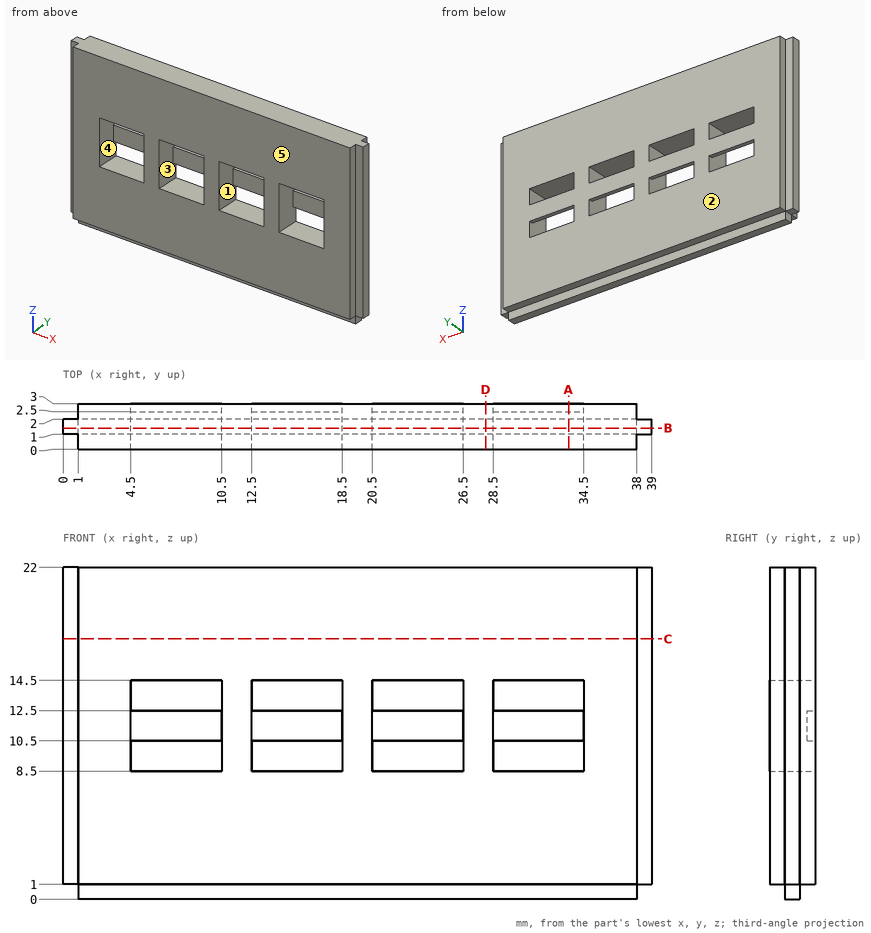
Here's the drawing with two shaded views (mm, measured from the low corner). I have some questions. A direction names the side the tool comes from. Coordinates: 2 decimals unless noted, no trailing zeros. Order: outer loops, then holes, each group sorted by start corner. A loop starts at its lowest first (then second) coordinate and runs counter-clockwise, first axis right, second up.
Q1. Suppose I cut it at C-C on z = 17.25. Please give me the cut outline in (x, y).
Q2. Which directions (+Z, -Z, +X, -X, +Y, -Y) give clear straight access to the entire face, cutting with the end or side of a thin tool? Please do the marked faces 4 and 5.
Q3. Suppose I cut it at B-B on y = 1.4. Please give me the cut outline in (x, z).
Q4. Please list where these lines run through material, in increasing order: L1, parallel to X at y = 1.4, z = 12; L2, parallel to Z at x = 30, y = 2.2; L3, parallel to Z at x = 34, y = 1.3.
Q5. Thinking about a two-plate mould opening in X: for the marked faces 1, 2 and 3, which applies, released by +X, released by -X, zero draft, split by the parting line, or undercut?
Q6. Will these pins go through, and if not, where does the flat tip stop? pin 1 (1.6 mm diameter, centred on x = 6.5, z = 11.5, fed in from -Y); pin 2 (0.6 mm diameter, centred on x = 8.5, y = 3, fed in from -Z); pin 3 (0.8 mm diameter, centred on y = 0.5, z = 12, fed in from +X).
Q7. Suppose I cut it at A-A on x = 33.5. Please give me the cut outline in (y, z).
Q8. Suppose I cut it at D-D on x = 28. Please give me the cut outline in (y, z).
Answer:
1. outline: (0, 1) - (1, 1) - (1, 0) - (38, 0) - (38, 1) - (39, 1) - (39, 2) - (38, 2) - (38, 3) - (1, 3) - (1, 2) - (0, 2) - close
2. face 4: -Y
2. face 5: +Z, -Z, +X, -X, -Y
3. outline: (0, 1) - (1, 1) - (1, 0) - (38, 0) - (38, 1) - (39, 1) - (39, 22) - (0, 22) - close; hole (4.5, 8.5) - (10.5, 8.5) - (10.5, 14.5) - (4.5, 14.5) - close; hole (12.5, 8.5) - (18.5, 8.5) - (18.5, 14.5) - (12.5, 14.5) - close; hole (20.5, 8.5) - (26.5, 8.5) - (26.5, 14.5) - (20.5, 14.5) - close; hole (28.5, 8.5) - (34.5, 8.5) - (34.5, 14.5) - (28.5, 14.5) - close
4. L1: x = 0 to 4.5, 10.5 to 12.5, 18.5 to 20.5, 26.5 to 28.5, 34.5 to 39
4. L2: z = 1 to 8.5, 14.5 to 22
4. L3: z = 0 to 8.5, 14.5 to 22
5. face 1: undercut
5. face 2: zero draft
5. face 3: undercut
6. pin 1: stops at y = 2.5
6. pin 2: stops at z = 1
6. pin 3: stops at x = 38
7. outline: (0, 1) - (1, 1) - (1, 0) - (2, 0) - (2, 1) - (3, 1) - (3, 8.5) - (0, 8.5) - close; (0, 14.5) - (3, 14.5) - (3, 22) - (0, 22) - close; (2.5, 10.5) - (3, 10.5) - (3, 12.5) - (2.5, 12.5) - close
8. outline: (0, 1) - (1, 1) - (1, 0) - (2, 0) - (2, 1) - (3, 1) - (3, 22) - (0, 22) - close
